Check sheet for the modelled part. Datum: model origin and axes. Units: mm. Face numbers are marked on the shaded views. A direction names the side the tool comes from. Coordinates: 2 decimals unless noted, no trailing zeros. Loops run counter-clockwise (first coordinate to the right, second up) from the corner with the lowest first, then second, coordinate; pieces in that order, holes last. Notation, with made-up numbers: M 26,-20.5 L 61,-20.5 A15 ccw 61,2.5 Z; hole C 38.5,53.5 d7. An arc over 180 degrees is marked long. Write each question's results on one line, items separated by ' | '. Start each with the question number.
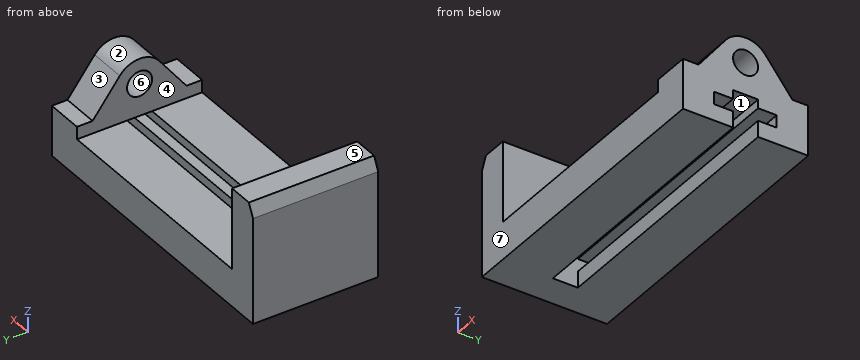
from build123d import *

# Parameters (mm, degrees)
F0_W     = 38.1
F0_H     = 41.149566
F1_DEPTH = 127
F3_DEPTH = 273.05
F2_R     = 12.7
F4_DEPTH = 254


with BuildPart() as f1:
    # F0 (on Front) → F1 (new body)
    with BuildSketch(Plane.XZ):
        Polygon((6.213259, 120.18176), (0, 107.315989), (0, 0), (304.8, 0), (304.8, 60.450434), (266.7, 60.450434), (266.7, 38.1), (31.75, 38.1), (31.75, 120.18176), align=None)
        with Locations((285.75, 81.025217)):
            Rectangle(F0_W, F0_H)
    extrude(amount=F1_DEPTH)

    # F2 (on face) → F3 (cut)
    with BuildSketch(Plane.YZ.offset(304.8)):
        Polygon((-76.2, 16.51), (-76.2, 0), (-50.8, 0), (-50.8, 16.51), (-31.905102, 16.51), (-31.905102, 29.21), (-50.8, 29.21), (-50.8, 38.1), (-76.2, 38.1), (-76.2, 29.21), (-95.405102, 29.21), (-95.405102, 16.51), align=None)
    extrude(amount=-F3_DEPTH, mode=Mode.SUBTRACT)

    # F2 (on face) → F4 (cut)
    with BuildSketch(Plane.YZ.offset(304.8)):
        with Locations((-63.5, 70.793197)):
            Circle(F2_R)
        with BuildLine():
            Line((-127, 101.6), (-127, 50.8))
            Line((-127, 50.8), (-111.125, 50.8))
            Line((-111.125, 50.8), (-83.577839, 86.350843))
            ThreePointArc((-83.577839, 86.350843), (-63.5, 96.193197), (-43.422161, 86.350843))
            Line((-43.422161, 86.350843), (-15.875, 50.8))
            Line((-15.875, 50.8), (0, 50.8))
            Line((0, 50.8), (0, 101.6))
            Line((0, 101.6), (-127, 101.6))
        make_face()
    extrude(amount=-F4_DEPTH, mode=Mode.SUBTRACT)


solid = f1.part
1) Section check A-A (x = 249). Enter the section's corners in (y, z), then the cut area to 3 significant figures.
2) Section check B-B (y = -63.5). Enter the section's corners in (x, z).
3) Thickness scan on probe 1 along Z at (x, y) = (238, -89.5); probe 2 along X at (y, z) = (-66.5, 57); probe 3 along Y at (x, z) = (147, 15.5). Record the ranges inside material, lowest first.
4) Set-up check for the marked faces 1, 2, 3 and 4: record each of +Z, -Z, +X, -X, +Y, -Y from which the full face is reachable in a straight line by a thin tool's end or side.
5) Section check C-C (z = 23.5). Enter the section's corners in (x, y), then the cut area to 3 significant figures.
6) Release check for a two-part mould opening along Z. For the marked faces 5, 6 and 7 record: +Z half, -Z half, draft (parallel to the pull), parting line (faces both ways), or undercut.
7) Gauge pin test, flat ends, axial feed: P1, Ø8, axis at x = 282, y = -4.5, coming from the +Z side; P2, Ø5, axis at x = 220.5, y = -106, coming from the +Z side; P3, Ø8, axis at x = 114.5, y = -33, coming from the -Z side; P4, Ø12, axis at y = -99.5, z = 78, coming from the +X side. Record the tip position at first contact, or that the pin passes through.
8) Section check D-D (z = 46). Enter the section's corners in (x, y).
Return value:
1) outline: M -127,0 L -76.2,0 L -76.2,16.51 L -95.41,16.51 L -95.41,29.21 L -76.2,29.21 L -76.2,38.1 L -127,38.1 Z; M -50.8,0 L 0,0 L 0,38.1 L -50.8,38.1 L -50.8,29.21 L -31.91,29.21 L -31.91,16.51 L -50.8,16.51 Z | area: 3,390 mm2
2) outline: M 0,0 L 31.75,0 L 31.75,120.18 L 6.21,120.18 L 0,107.32 Z; M 266.7,38.1 L 304.8,38.1 L 304.8,58.09 L 266.7,58.09 Z; M 266.7,83.49 L 304.8,83.49 L 304.8,96.19 L 266.7,96.19 Z
3) probe 1: z = 0 to 16.51, 29.21 to 38.1 | probe 2: x = 0 to 31.75, 266.7 to 304.8 | probe 3: y = -127 to -76.2, -50.8 to 0
4) face 1: -Z, +X | face 2: +Z, +X | face 3: +Z, +X, +Y | face 4: +Z, +Y, -Y
5) outline: M 0,-127 L 304.8,-127 L 304.8,-95.41 L 31.75,-95.41 L 31.75,-31.91 L 304.8,-31.91 L 304.8,0 L 0,0 Z | area: 21,400 mm2
6) face 5: +Z half | face 6: undercut | face 7: draft
7) P1: stops at z = 50.8 | P2: stops at z = 38.1 | P3: stops at z = 0 | P4: stops at x = 31.75
8) outline: M 0,-127 L 31.75,-127 L 31.75,0 L 0,0 Z; M 266.7,-127 L 304.8,-127 L 304.8,0 L 266.7,0 Z
